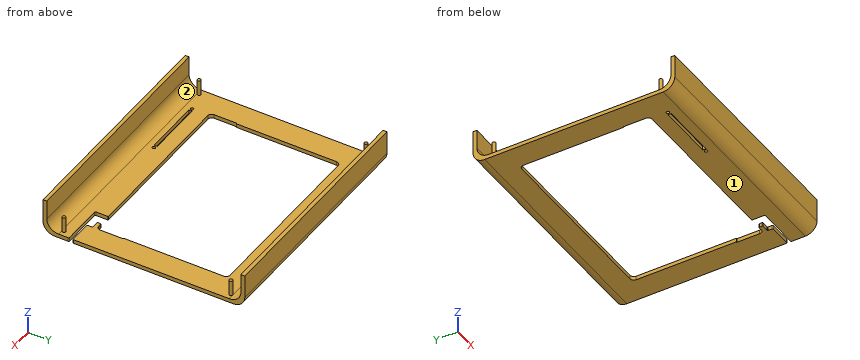
Autodesk Fusion 360 part; units mm, degrees
sketch "Sketch1" plane through (0, 0, 0) normal (0, 0, 1) x (1, 0, 0)
  line L0 (0, 0) -> (300, 0)
  line L1 (300, 0) -> (300, 260)
  line L2 (300, 260) -> (0, 260)
  line L3 (0, 260) -> (0, 0)
  circle A0 centre (7.5, 22.5) radius 2.25
  circle A1 centre (292.5, 22.5) radius 2.25
  circle A2 centre (7.5, 237.5) radius 2.25
  circle A3 centre (292.5, 237.5) radius 2.25
  dimension "d1" = 300
  dimension "d2" = 260
  dimension "d3" = 4.5
  dimension "d4" = 4.5
  dimension "d5" = 4.5
  dimension "d6" = 4.5
  dimension "d7" = 22.5
  dimension "d8" = 7.5
  dimension "d9" = 22.5
  dimension "d10" = 7.5
  dimension "d11" = 7.5
  dimension "d12" = 22.5
  dimension "d13" = 22.5
  dimension "d14" = 7.5
extrude "Extrude1" add sketch "Sketch1" along normal blind 5
extrude "Extrude2" add sketch "Sketch1" along normal blind 25 contours A0
extrude "Extrude3" add sketch "Sketch1" along normal blind 25 contours A2
extrude "Extrude4" add sketch "Sketch1" along normal blind 25 contours A3
extrude "Extrude5" add sketch "Sketch1" along normal blind 25 contours A1
sketch "Sketch2" plane through (0, 0, 5) normal (0, 0, 1) x (-1, 0, 0)
  circle A0 centre (-7.5, -22.5) radius 2.25
  circle A1 centre (-7.5, -237.5) radius 2.25
  circle A2 centre (-292.5, -22.5) radius 2.25
  circle A3 centre (-292.5, -237.5) radius 2.25
  line L0 (0, -260) -> (0, 0)
  line L1 (0, 0) -> (-300, 0)
  line L2 (-300, 0) -> (-300, -260)
  line L3 (-300, -260) -> (0, -260)
  line L4 (-30, -220) -> (-270, -220)
  line L5 (-270, -220) -> (-270, -55.5)
  line L6 (-270, -50.5) -> (-30, -50.5)
  line L7 (-30, -50.5) -> (-30, -220)
  line L8 (-300, -260) -> (0, -260)
  line L9 (0, 0) -> (-300, 0)
  line L10 (0, -260) -> (0, 0)
  line L11 (-300, 0) -> (-300, -260)
  line L12 (-30, -220) -> (-270, -220)
  line L13 (-270, -220) -> (-270, -219)
  line L14 (-270, -219) -> (-30, -219)
  line L15 (-30, -219) -> (-30, -220)
  line L16 (-270, -220) -> (-269, -220)
  line L17 (-269, -220) -> (-269, -85)
  line L18 (-269, -85) -> (-270, -85)
  line L19 (-270, -85) -> (-270, -220)
  line L20 (-30, -220) -> (-31, -220)
  line L21 (-31, -220) -> (-31, -85)
  line L22 (-31, -85) -> (-30, -85)
  line L23 (-30, -85) -> (-30, -220)
  line L24 (-36, -219) -> (-36, -219)
  line L25 (-36, -219) -> (-36, -214)
  line L26 (-36, -214) -> (-31, -214)
  line L27 (-31, -214) -> (-31, -214)
  arc A4 (-36, -219) -> (-31, -214) centre (-36, -214) ccw
  line L28 (-264, -219) -> (-264, -219)
  line L29 (-264, -219) -> (-264, -214)
  line L30 (-264, -214) -> (-269, -214)
  line L31 (-269, -214) -> (-269, -214)
  arc A5 (-269, -214) -> (-264, -219) centre (-264, -214) ccw
  line L32 (-265, -50.5) -> (-265, -50.5)
  line L33 (-265, -50.5) -> (-265, -55.5)
  line L34 (-265, -55.5) -> (-270, -55.5)
  line L35 (-270, -55.5) -> (-270, -50.5)
  arc A6 (-265, -50.5) -> (-270, -55.5) centre (-265, -55.5) ccw
  line L36 (-35, -50.5) -> (-35, -50.5)
  line L37 (-35, -50.5) -> (-35, -55.5)
  line L38 (-35, -55.5) -> (-30, -55.5)
  line L39 (-30, -55.5) -> (-30, -55.5)
  arc A7 (-30, -55.5) -> (-35, -50.5) centre (-35, -55.5) ccw
  point P0 (-31, -219)
  point P1 (-269, -219)
  dimension "d25" = 240
  dimension "d26" = 169.5
  dimension "d27" = 40
  dimension "d28" = 50.5
  dimension "d29" = 30
  dimension "d30" = 30
  dimension "d31" = 1
  dimension "d32" = 135
  dimension "d33" = 1
  dimension "d34" = 135
  dimension "d35" = 1
  dimension "d36" = 5
  dimension "d37" = 5
  dimension "d38" = 5
  dimension "d39" = 5
  dimension "d40" = 5
  dimension "d41" = 5
  dimension "d42" = 5
  dimension "d43" = 5
  dimension "d44" = 5
  dimension "d45" = 5
  dimension "d46" = 5
  dimension "d47" = 5
extrude "Extrude6" cut sketch "Sketch2" against normal blind 5 contours L5 L6 L7 L14 L17 L18 L21 L22 L25 L26 L29 L30 L33 L34 L37 L38
extrude "Extrude7" cut sketch "Sketch2" against normal blind 5 contours L37 L38 A7
extrude "Extrude8" cut sketch "Sketch2" against normal blind 5 contours L33 L34 A6
extrude "Extrude9" cut sketch "Sketch2" against normal blind 5 contours L29 L30 A5
extrude "Extrude10" cut sketch "Sketch2" against normal blind 5 contours L25 L26 A4
sketch "Sketch3" plane through (0, 0, 5) normal (0, 0, 1) x (-1, 0, 0)
  arc A0 (-36, -219) -> (-31, -214) centre (-36, -214) ccw
  line L0 (-36, -219) -> (-264, -219)
  arc A1 (-269, -214) -> (-264, -219) centre (-264, -214) ccw
  line L1 (-269, -214) -> (-269, -85)
  line L2 (-269, -85) -> (-270, -85)
  line L3 (-270, -85) -> (-270, -55.5)
  arc A2 (-265, -50.5) -> (-270, -55.5) centre (-265, -55.5) ccw
  line L4 (-265, -50.5) -> (-35, -50.5)
  arc A3 (-30, -55.5) -> (-35, -50.5) centre (-35, -55.5) ccw
  line L5 (-30, -55.5) -> (-30, -85)
  line L6 (-30, -85) -> (-31, -85)
  line L7 (-31, -85) -> (-31, -214)
  line L8 (0, -260) -> (0, 0)
  line L9 (0, 0) -> (-300, 0)
  line L10 (-300, 0) -> (-300, -260)
  line L11 (-300, -260) -> (0, -260)
  circle A4 centre (-292.5, -237.5) radius 2.25
  circle A5 centre (-292.5, -22.5) radius 2.25
  circle A6 centre (-7.5, -237.5) radius 2.25
  circle A7 centre (-7.5, -22.5) radius 2.25
  line L12 (0, 0) -> (-300, 0)
  line L13 (-300, 0) -> (-300, -5)
  line L14 (-300, -5) -> (0, -5)
  line L15 (0, -5) -> (0, 0)
  line L16 (0, -260) -> (-300, -260)
  line L17 (-300, -260) -> (-300, -255)
  line L18 (-300, -255) -> (0, -255)
  line L19 (0, -255) -> (0, -260)
  dimension "d58" = 300
  dimension "d59" = 5
  dimension "d60" = 300
  dimension "d61" = 5
extrude "Extrude11" add sketch "Sketch3" along normal blind 40 contours L8 L10 L11 L16 L17 L18 L19
extrude "Extrude12" add sketch "Sketch3" along normal blind 40 contours L8 L9 L10 L12 L13 L14 L15
fillet "Fillet1" radius 15 1 edges at (150, 255, 5)
fillet "Fillet2" radius 15 1 edges at (150, 260, 0)
fillet "Fillet3" radius 15 1 edges at (150, 5, 5)
fillet "Fillet4" radius 15 1 edges at (150, 0, 0)
sketch "Sketch4" plane through (0, 0, 0) normal (0, 0, -1) x (1, 0, 0)
  line L0 (300, -15) -> (0, -15)
  line L1 (0, -15) -> (0, -245)
  line L2 (0, -245) -> (300, -245)
  line L3 (300, -245) -> (300, -15)
  arc A0 (31, -214) -> (36, -219) centre (36, -214) ccw
  line L4 (31, -214) -> (31, -85)
  line L5 (31, -85) -> (30, -85)
  line L6 (30, -85) -> (30, -55.5)
  arc A1 (35, -50.5) -> (30, -55.5) centre (35, -55.5) ccw
  line L7 (35, -50.5) -> (265, -50.5)
  arc A2 (270, -55.5) -> (265, -50.5) centre (265, -55.5) ccw
  line L8 (270, -55.5) -> (270, -85)
  line L9 (270, -85) -> (269, -85)
  line L10 (269, -85) -> (269, -214)
  arc A3 (264, -219) -> (269, -214) centre (264, -214) ccw
  line L11 (264, -219) -> (36, -219)
  line L12 (245, -50.5) -> (260, -50.5)
  line L13 (260, -50.5) -> (260, -33.5)
  line L14 (260, -33.5) -> (245, -33.5)
  line L15 (245, -33.5) -> (245, -50.5)
  line L16 (260, -33.5) -> (270, -33.5)
  line L17 (270, -33.5) -> (270, -45.5)
  line L18 (270, -45.5) -> (260, -45.5)
  line L19 (260, -45.5) -> (260, -33.5)
  line L20 (270, -33.5) -> (300, -33.5)
  line L21 (300, -33.5) -> (300, -38.5)
  line L22 (300, -38.5) -> (270, -38.5)
  line L23 (270, -38.5) -> (270, -33.5)
  dimension "d74" = 15
  dimension "d75" = 17
  dimension "d76" = 10
  dimension "d77" = 12
  dimension "d78" = 30
  dimension "d79" = 30
  dimension "d80" = 5
extrude "Extrude13" cut sketch "Sketch4" against normal blind 5 contours L7 L12 L13 L14 L15 L19
extrude "Extrude14" cut sketch "Sketch4" against normal blind 5 contours L13 L16 L17 L18 L19 L23
extrude "Extrude15" cut sketch "Sketch4" against normal blind 5 contours L3 L17 L20 L21 L22 L23
fillet "Fillet5" radius 1 1 edges at (245, 50.5, 2.5)
fillet "Fillet6" radius 1 1 edges at (245, 33.5, 2.5)
fillet "Fillet7" radius 1 1 edges at (260, 50.5, 2.5)
fillet "Fillet8" radius 1 1 edges at (260, 45.5, 2.5)
fillet "Fillet9" radius 1 1 edges at (270, 45.5, 2.5)
fillet "Fillet10" radius 1 1 edges at (270, 38.5, 2.5)
fillet "Fillet11" radius 1 1 edges at (300, 33.5, 2.5)
fillet "Fillet12" radius 1 1 edges at (300, 38.5, 2.5)
sketch "Sketch5" plane through (0, 0, 0) normal (0, 0, -1) x (1, 0, 0)
  arc A0 (300, -39.5) -> (299, -38.5) centre (299, -39.5) ccw
  line L0 (299, -38.5) -> (271, -38.5)
  arc A1 (271, -38.5) -> (270, -39.5) centre (271, -39.5) ccw
  line L1 (270, -39.5) -> (270, -44.5)
  arc A2 (269, -45.5) -> (270, -44.5) centre (269, -44.5) ccw
  line L2 (269, -45.5) -> (261, -45.5)
  arc A3 (261, -45.5) -> (260, -46.5) centre (261, -46.5) ccw
  line L3 (260, -46.5) -> (260, -49.5)
  arc A4 (260, -49.5) -> (261, -50.5) centre (261, -49.5) ccw
  line L4 (261, -50.5) -> (265, -50.5)
  arc A5 (270, -55.5) -> (265, -50.5) centre (265, -55.5) ccw
  line L5 (270, -55.5) -> (270, -85)
  line L6 (270, -85) -> (269, -85)
  line L7 (269, -85) -> (269, -214)
  arc A6 (264, -219) -> (269, -214) centre (264, -214) ccw
  line L8 (264, -219) -> (36, -219)
  arc A7 (31, -214) -> (36, -219) centre (36, -214) ccw
  line L9 (31, -214) -> (31, -85)
  line L10 (31, -85) -> (30, -85)
  line L11 (30, -85) -> (30, -55.5)
  arc A8 (35, -50.5) -> (30, -55.5) centre (35, -55.5) ccw
  line L12 (35, -50.5) -> (244, -50.5)
  arc A9 (244, -50.5) -> (245, -49.5) centre (244, -49.5) ccw
  line L13 (245, -49.5) -> (245, -34.5)
  arc A10 (246, -33.5) -> (245, -34.5) centre (246, -34.5) ccw
  line L14 (246, -33.5) -> (299, -33.5)
  arc A11 (299, -33.5) -> (300, -32.5) centre (299, -32.5) ccw
  line L15 (300, -32.5) -> (300, -15)
  line L16 (300, -15) -> (0, -15)
  line L17 (0, -15) -> (0, -245)
  line L18 (0, -245) -> (300, -245)
  line L19 (300, -245) -> (300, -39.5)
  line L20 (30, -23.5) -> (118, -23.5)
  line L21 (118, -23.5) -> (118, -35.5)
  line L22 (118, -35.5) -> (30, -35.5)
  line L23 (30, -35.5) -> (30, -23.5)
  line L24 (37.5, -27.5) -> (110.5, -27.5)
  line L25 (110.5, -27.5) -> (110.5, -31.5)
  line L26 (110.5, -31.5) -> (37.5, -31.5)
  line L27 (37.5, -31.5) -> (37.5, -27.5)
  circle A12 centre (114.25, -29.5) radius 1.95
  circle A13 centre (33.75, -29.5) radius 1.95
  dimension "d103" = 88
  dimension "d104" = 12
  dimension "d105" = 15
  dimension "d106" = 30
  dimension "d107" = 73
  dimension "d108" = 4
  dimension "d109" = 4
  dimension "d110" = 7.5
  dimension "d111" = 3.9
  dimension "d112" = 3.75
  dimension "d113" = 3.9
  dimension "d114" = 3.75
  dimension "d115" = 6
  dimension "d116" = 6
extrude "Extrude16" cut sketch "Sketch5" against normal blind 5 contours L24 L25 L26 L27
extrude "Extrude17" cut sketch "Sketch5" against normal blind 5 contours A13
extrude "Extrude18" cut sketch "Sketch5" against normal blind 5 contours A12
Can you work these out from the model? Positions are in its coordinate system, mm. Face numbers are marked on the shaded views. A direction names the side the tool comes from. Give positions to 0.01 mm unless a question says otherwise; leave off trailing zeros. Loops run counter-clockwise (first coordinate to the right, second up) from the corner with the lowest first, then second, coordinate; pieces in that order, holes last. Notation, with made-up numbers: (61, -14.5) - (83, -14.5) arc R24 ccw to (83, 22.5) - close; hole circle Ø6 at (-17, -35). An arc over 180 degrees is marked (long way). One line per item, written item: value.
(1) I need wall thicknesses on line 1 along X through (y, z) = (29.5, 1); line 2 along Y through (x, z) = (222, 42); line 3 along X through (y, z) = (95, 4.5). Which ranges of each line are inside material? Lowest first, please.
Verdict:
line 1: 0 to 31.8, 35.7 to 37.5, 110.5 to 112.3, 116.2 to 300
line 2: 0 to 5, 255 to 260
line 3: 0 to 31, 269 to 300
(2) On a 3-axis mill with a long thin cutter (end or side, diameter ignored), from which of +Z, -Z, +X, -X, +Y, -Y can I reach the whole of each face in a straight line? I mean the marked faces 1 and 2. Say none if no direction works.
Verdict:
face 1: -Z, +X, -X, +Y, -Y
face 2: +Z, +X, -X
(3) I'm going to push flat-ended pins straight in: pin 1 (0.5 mm diameter, centred on x = 269.5, z = 3.5, fed in from -Y); pin 2 (1.5 mm diameter, centred on x = 245.5, y = 50, fed in from +Z); pin 3 (3.5 mm diameter, centred on x = 291.5, y = 22.5, fed in from +Z). Where does each tip first touch, or does it pass through?
Verdict:
pin 1: y = 5.08
pin 2: z = 5
pin 3: z = 25
(4) If we section it at A-A, the plane x = 99: List the corners of the cut face in (y, z) for me.
Verdict:
outline: (0, 15) arc R15 ccw to (15, 0) - (27.5, 0) - (27.5, 5) - (20, 5) arc R15 cw to (5, 20) - (5, 45) - (0, 45) - close; (31.5, 0) - (50.5, 0) - (50.5, 5) - (31.5, 5) - close; (219, 0) - (245, 0) arc R15 ccw to (260, 15) - (260, 45) - (255, 45) - (255, 20) arc R15 cw to (240, 5) - (219, 5) - close
(5) If we section it at D-D, the plane z = 31.5: List the corners of the cut face in (x, y) for me, plus the area to 3 significant figures.
Verdict:
outline: (0, 0) - (300, 0) - (300, 5) - (0, 5) - close; (0, 255) - (300, 255) - (300, 260) - (0, 260) - close
area: 3,000 mm^2
(6) If we section it at B-B, the plane y = 80: List the corners of the cut face in (x, z) for me.
Verdict:
outline: (0, 0) - (30, 0) - (30, 5) - (0, 5) - close; (270, 0) - (300, 0) - (300, 5) - (270, 5) - close
(7) If we section it at C-C, the plane x = 214.5: List the corners of the cut face in (y, z) for me.
Verdict:
outline: (0, 15) arc R15 ccw to (15, 0) - (50.5, 0) - (50.5, 5) - (20, 5) arc R15 cw to (5, 20) - (5, 45) - (0, 45) - close; (219, 0) - (245, 0) arc R15 ccw to (260, 15) - (260, 45) - (255, 45) - (255, 20) arc R15 cw to (240, 5) - (219, 5) - close
